Part model, mm, in its own coordinate system. A direction names the side the tool comes from. Coordinates: 2 decimals unless noted, no trailing zeros. Write each loop counter-clockwise with the first axis right and the second up, starting at its lowest first coordinate (ties: lowest second). Pieces come first, ordered by that corner, then holes. Notation, with made-up numbers: (67, 30) -> (108, 30) arc R27 ccw to (108, 59) -> close; hole circle Ø7 at (28.5, -34.5). An arc over 180 degrees is marked (long way). Write item = value, one per line.
from build123d import *

# Parameters (mm, degrees)
F0_W     = 58
F0_H     = 23
F0_R     = 1.5
F1_DEPTH = 2.5
F2_W     = 24
F2_H     = 2.8
F3_DEPTH = 6.5


with BuildPart() as f1:
    # F0 (on Top) → F1 (new body)
    with BuildSketch(Plane.XY):
        Rectangle(F0_W, F0_H)
        with Locations((-25, -9)):
            Circle(F0_R, mode=Mode.SUBTRACT)
        with Locations((25, -9)):
            Circle(F0_R, mode=Mode.SUBTRACT)
    extrude(amount=F1_DEPTH)

    # F2 (on face) → F3 (join)
    with BuildSketch(Plane.XY.offset(2.5)):
        with Locations((0, 7)):
            Rectangle(F2_W, F2_H)
    extrude(amount=F3_DEPTH)


solid = f1.part
Q1. Saw through at B-B on y = -9. Give the cut face in (x, z).
Model answer:
outline = (-29, 0) -> (-26.5, 0) -> (-26.5, 2.5) -> (-29, 2.5) -> close; (-23.5, 0) -> (23.5, 0) -> (23.5, 2.5) -> (-23.5, 2.5) -> close; (26.5, 0) -> (29, 0) -> (29, 2.5) -> (26.5, 2.5) -> close
Q2. Mould opens along Y. For faces 5 (the face through (23.5, -8.93, 1.23)), 6 (the face through (0, 11.5, 1)), 7 (the face through (-12, 7, 6)), 8 (the face through (-26.5, -8.93, 1.23)) say: released by +Y, released by -Y, zero draft, split by the parting line, or undercut.
Model answer:
face_5 = undercut
face_6 = released by +Y
face_7 = zero draft
face_8 = undercut
Q3. Probe line 1 (Y direction, x = -25, z = 0.55); line 2 (Z direction, x = -15.5, y = 5); line 3 (Y direction, x = 8, z = 4.5). List the from-to ranges inside material, lowest first. Write a range as from..to.
Model answer:
line_1 = -11.5..-10.5, -7.5..11.5
line_2 = 0..2.5
line_3 = 5.6..8.4
Q4. Which spindle directions (+Z, -Z, +X, -X, +Y, -Y) get a long thin tool onto all of the face, cutting with end or side? Do faces 1 (the face through (0, 8.4, 6)), 2 (the face through (0, 5.6, 6)), 3 (the face through (0, -11.5, 1)), 4 (the face through (12, 7, 6)). Say none if no direction does.
Model answer:
face_1 = +Z, +X, -X, +Y
face_2 = +Z, +X, -X, -Y
face_3 = +Z, -Z, +X, -X, -Y
face_4 = +Z, +X, +Y, -Y
Q5. Saw through at D-D on z = 3.75. Give the cut face in (x, y).
Model answer:
outline = (-12, 5.6) -> (12, 5.6) -> (12, 8.4) -> (-12, 8.4) -> close
Q6. Saw through at A-A on x = 25. Give the cut face in (y, z).
Model answer:
outline = (-11.5, 0) -> (-10.5, 0) -> (-10.5, 2.5) -> (-11.5, 2.5) -> close; (-7.5, 0) -> (11.5, 0) -> (11.5, 2.5) -> (-7.5, 2.5) -> close
Q7. Pin check, flat tips, straight feed: pin 1 (3 mm diameter, centred on y = 7, z = 5.5, fed in from -X); pin 2 (2.5 mm diameter, centred on x = -25, y = -9, fed in from -Z); pin 3 (2 mm diameter, centred on y = 7.5, z = 6, fed in from +X); pin 4 (2 mm diameter, centred on x = 0.5, z = 6.5, fed in from -Y). Stop position of each tip, or through.
Model answer:
pin_1 = -12
pin_2 = through
pin_3 = 12
pin_4 = 5.6
Q8. Saw through at C-C on x = -10. Give the cut face in (y, z).
Model answer:
outline = (-11.5, 0) -> (11.5, 0) -> (11.5, 2.5) -> (8.4, 2.5) -> (8.4, 9) -> (5.6, 9) -> (5.6, 2.5) -> (-11.5, 2.5) -> close
